```python
from build123d import *


with BuildPart() as part:
    # Sketch1 → Revolve1 (revolve)
    with BuildSketch(Plane.XY):
        with BuildLine():
            Line((0, 3.5), (0, 2.65))
            ThreePointArc((0, 2.65), (0.043933983, 2.543933983), (0.15, 2.5))
            Line((0.15, 2.5), (3.85, 2.5))
            ThreePointArc((3.85, 2.5), (3.956066017, 2.543933983), (4, 2.65))
            Line((4, 2.65), (4, 3.5))
            Line((4, 3.5), (3.8345, 3.5))
            Line((3.8345, 3.5), (3.8345, 4.65))
            Line((3.8345, 4.65), (4, 4.65))
            Line((4, 4.65), (4, 5.5))
            ThreePointArc((4, 5.5), (3.956066017, 5.606066017), (3.85, 5.65))
            Line((3.85, 5.65), (0.15, 5.65))
            ThreePointArc((0.15, 5.65), (0.043933983, 5.606066017), (0, 5.5))
            Line((0, 5.5), (0, 4.65))
            Line((0, 4.65), (0.1655, 4.65))
            Line((0.1655, 4.65), (0.1655, 3.5))
            Line((0.1655, 3.5), (0, 3.5))
        make_face()
    revolve(axis=Axis((-0.0025, 0, 0), (1, 0, 0)))


solid = part.part
```
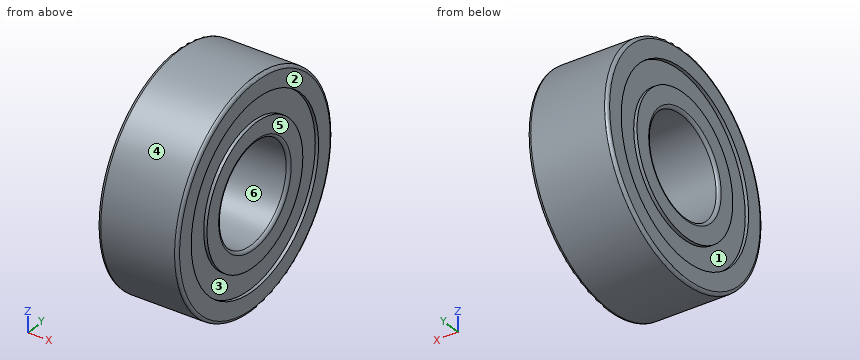
Part model, mm, in its own coordinate system. Face numbers are marked on the shaded views. A direction names the side the tool comes from. Round coordinates to 2 decimals unless told otherwise and drop trailing zeros. Write each loop counter-clockwise with the first axis right and the second up, starting at its lowest first coordinate (ties: lowest second). Pieces come first, ordered by that corner, then holes. Notation, with made-up numbers: (2, -7) -> (16, -7) arc R22 cw to (16, 8) -> close; hole circle Ø10 at (61, 70.25). An arc over 180 degrees is marked (long way). Return JSON: item names as keys, results as strings. Group by question number.
Q1. Probe L1, parallel to Z at x = 2.45, y = 0; L2, parallel to Z at x = 0.1, y = 0; L3, parallel to Y at x = 3.4, z = 0.25. List the from-to ranges inside material, lowest first. Write a range as [from, to].
Q2. Mould opens along Y. For the marked faces 4, 5 and 6 say: pulls with the +Y half, pulls with the -Y half, needs draft (parallel to the pull), parting line crosses it, or undercut.
Q3. Which spindle directions (+Z, -Z, +X, -X, +Y, -Y) get a long thin tool onto all of the face, cutting with end or side? Do the marked faces 1, 2 and 3. Say none if no direction does.
Q4. Saw through at C-C on x = 2.3. Write the cut outline in (y, z), plus the area to 3 significant figures.
Q5. Pin check, flat tips, straight feed: pin 1 (1.5 mm diameter, centred on x = 3.5, y = -1.5, fed in from +Z); pin 2 (1.5 mm diameter, centred on x = 1, z = -2, fed in from -Y). Stop position of each tip, or through.
Answer:
{
 "1": {"L1": "[-5.65, -2.5], [2.5, 5.65]", "L2": "[-5.64, -4.65], [-3.5, -2.51], [2.51, 3.5], [4.65, 5.64]", "L3": "[-5.64, -2.49], [2.49, 5.64]"},
 "2": {"face 4": "parting line crosses it", "face 5": "needs draft", "face 6": "undercut"},
 "3": {"face 1": "-X", "face 2": "+Z, -Z, +X, +Y, -Y", "face 3": "+X"},
 "4": {"outline": "circle Ø11.3 at (0, 0); hole circle Ø5 at (0, 0)", "area": "80.7 mm2"},
 "5": {"pin 1": "z = 5.6", "pin 2": "y = -5.51"}
}
